Solid Edge part; units mm, degrees
sketch "Sketch1" plane through (0, 0, 0) normal (1, 0, 0) x (0, 1, 0)
  line L0 (0, 50.8) -> (0, 0)
  line L1 (0, 0) -> (25.4, 0)
  arc A0 (25.4, 0) -> (20.6248, 4.7752) centre (20.6248, 0) ccw
  line L2 (20.6248, 4.7752) -> (7.9502, 4.7752)
  arc A1 (7.9502, 4.7752) -> (4.7752, 7.9502) centre (7.9502, 7.9502) cw
  line L3 (4.7752, 7.9502) -> (4.7752, 46.0248)
  arc A2 (4.7752, 46.0248) -> (0, 50.8) centre (0, 46.0248) ccw
extrude "ExtrudedProtrusion_1" add sketch "Sketch1" against normal blind 36.5125 and the other way blind 36.5125
hole "Hole_1" at (25.4, 0, 12.7) direction (0, 1, 0) diameter 7.1374 depth 5.2527
hole "Hole_2" at (0, 0, 12.7) direction (0, 1, 0) diameter 7.1374 depth 5.2527
hole "Hole_3" at (-25.4, 0, 12.7) direction (0, 1, 0) diameter 7.1374 depth 5.2527
hole "Hole_4" at (25.4, 0, 38.1) direction (0, 1, 0) diameter 7.1374 depth 5.2527
hole "Hole_5" at (0, 0, 38.1) direction (0, 1, 0) diameter 7.1374 depth 5.2527
hole "Hole_6" at (-25.4, 0, 38.1) direction (0, 1, 0) diameter 7.1374 depth 5.2527
sketch "Sketch2" plane through (0, 0, 0) normal (0, 0, 1) x (1, 0, 0)
  arc A0 (21.8313, 12.7) -> (28.9687, 12.7) centre (25.4, 12.7) ccw
  line L0 (28.9687, 12.7) -> (28.9687, 17.4752)
  arc A1 (28.9687, 17.4752) -> (21.8313, 17.4752) centre (25.4, 17.4752) ccw
  line L1 (21.8313, 17.4752) -> (21.8313, 12.7)
extrude "ExtrudedCutout_1" cut sketch "Sketch2" along normal blind 7.1628
sketch "Sketch3" plane through (0, 0, 0) normal (0, 0, 1) x (1, 0, 0)
  arc A0 (-3.5687, 12.7) -> (3.5687, 12.7) centre (0, 12.7) ccw
  line L0 (3.5687, 12.7) -> (3.5687, 17.4752)
  arc A1 (3.5687, 17.4752) -> (-3.5687, 17.4752) centre (0, 17.4752) ccw
  line L1 (-3.5687, 17.4752) -> (-3.5687, 12.7)
extrude "ExtrudedCutout_2" cut sketch "Sketch3" along normal blind 7.1628
sketch "Sketch4" plane through (0, 0, 0) normal (0, 0, 1) x (1, 0, 0)
  arc A0 (-28.9687, 12.7) -> (-21.8313, 12.7) centre (-25.4, 12.7) ccw
  line L0 (-21.8313, 12.7) -> (-21.8313, 17.4752)
  arc A1 (-21.8313, 17.4752) -> (-28.9687, 17.4752) centre (-25.4, 17.4752) ccw
  line L1 (-28.9687, 17.4752) -> (-28.9687, 12.7)
extrude "ExtrudedCutout_3" cut sketch "Sketch4" along normal blind 7.1628
properties part number "4251"
Here's how the part is built. I have some questions about the finished solid (model axes, mm). A direction names the side the tool comes from. Coordinates: 2 decimals unless noted, no trailing zeros. Write each loop counter-clockwise with the first axis right and the second up, starting at its lowest first coordinate (ties: lowest second). Pieces come first, ordered by that corner, then holes.
Item 1: I want a section at A-A on z = 12.7. Write out the boundary of the cut face in (x, y), and give its area (3 significant figures).
Item 2: If I drill on line 1 (X direction, y = 3.6, z = 38.1); line 2 (Z direction, x = 25.4, y = 1.65); line 3 (Y direction, x = -30.5, z = 15.5), over which ranges is the centre line in solid material (lowest first)?
Item 3: I want a section at B-B on x = 31.5. Write out the boundary of the cut face in (y, z) (3 decimals), and give its area (3 significant figures).
Item 4: On a 3-axis mill with a long thin cutter (end or side, diameter ignored), from which of +Z, -Z, +X, -X, +Y, -Y can I reach the whole of each face in a straight line? I mean faces 1 (the cylindrical face through (-1.072, 2.421, 34.696)), 2 (the flat face through (21.831, 15, 2)). Say none if no direction works.
Item 5: If we mould it in two halves opening along Z, with no side actions, what happens to faces 3 (the cylindrical face through (-28.41, 2.42, 36.18)), 4 (the flat face through (-3.569, 15, 2)), 5 (the cylindrical face through (0.51, 24.04, 3.34))? For each: +Z half, -Z half, draft (parallel to the pull), parting line (faces both ways), or undercut.
Item 6: I want a section at D-D on x = 0. Write out the boundary of the cut face in (y, z) (3 decimals).
Item 7: I want a section at C-C on y = 3. Write out the boundary of the cut face in (x, z).
Item 8: Will these pins go through, and if not, where does the flat tip stop? pin 1 (2 mm diameter, centred on x = 7, z = 11.5, fed in from +Y); pin 2 (5 mm diameter, centred on x = 7.5, y = 14, fed in from +Z); pin 3 (11.5 mm diameter, centred on x = -25.4, z = 12.7, fed in from +Y).
Findings below:
1. outline: (-36.51, 0) - (-28.97, 0) - (-28.97, 4.78) - (-36.51, 4.78) - close; (-21.83, 0) - (-3.57, 0) - (-3.57, 4.78) - (-21.83, 4.78) - close; (3.57, 0) - (21.83, 0) - (21.83, 4.78) - (3.57, 4.78) - close; (28.97, 0) - (36.51, 0) - (36.51, 4.78) - (28.97, 4.78) - close
1. area: 246 mm2
2. line 1: x = -36.51 to -28.97, -21.83 to -3.57, 3.57 to 21.83, 28.97 to 36.51
2. line 2: z = 0 to 9.13, 16.27 to 34.53, 41.67 to 50.51
2. line 3: y = 0 to 4.78
3. outline: (0, 0) - (25.4, 0) arc R4.775 ccw to (20.625, 4.775) - (7.95, 4.775) arc R3.175 cw to (4.775, 7.95) - (4.775, 46.025) arc R4.775 ccw to (0, 50.8) - close
3. area: 333 mm2
4. face 1: +Y, -Y
4. face 2: +Z, -Z
5. face 3: undercut
5. face 4: draft
5. face 5: +Z half
6. outline: (0, 0) - (9.131, 0) - (9.131, 4.775) - (7.95, 4.775) arc R3.175 cw to (4.775, 7.95) - (4.775, 9.131) - (0, 9.131) - close; (0, 16.269) - (4.775, 16.269) - (4.775, 34.531) - (0, 34.531) - close; (0, 41.669) - (4.775, 41.669) - (4.775, 46.025) arc R4.775 ccw to (0, 50.8) - close; (21.044, 0) - (25.4, 0) arc R4.775 ccw to (21.044, 4.757) - close
7. outline: (-36.51, 0) - (36.51, 0) - (36.51, 49.74) - (-36.51, 49.74) - close; hole circle Ø7.14 at (-25.4, 12.7); hole circle Ø7.14 at (-25.4, 38.1); hole circle Ø7.14 at (0, 12.7); hole circle Ø7.14 at (0, 38.1); hole circle Ø7.14 at (25.4, 12.7); hole circle Ø7.14 at (25.4, 38.1)
8. pin 1: stops at y = 4.78
8. pin 2: stops at z = 4.78
8. pin 3: stops at y = 4.94
